The listing builds one solid part. Answer for the finished solid, in the listing's coordinates (mm). Coordinates: 2 decimals unless noted, no trailing zeros. Order: outer loops, then holes, each group sorted by start corner. A loop starts at its lowest first (then second) coordinate and runs counter-clockwise, first axis right, second up. Notation, with made-up numbers: (-29, -39) -> (23, -39) arc R35 cw to (23, -3) -> close; hole circle Ø8 at (-37, -37.5). An arc over 180 degrees is marked (long way). Return JSON: item names as keys, results as strings.
from build123d import *

# Parameters (mm, degrees)
F1_DEPTH = 6.5
F3_DEPTH = 80


with BuildPart() as f1:
    # F0 (on Front) → F1 (new body, symmetric)
    with BuildSketch(Plane.XZ):
        Polygon((80, 0), (0, 0), (0, -20), (80, -5), align=None)
    extrude(amount=F1_DEPTH, both=True)

    # F2 (on Right) → F3 (intersect)
    with BuildSketch(Plane.YZ):
        with BuildLine():
            Line((6.5, 0), (-6.5, 0))
            Line((-6.5, 0), (-6.5, -5))
            ThreePointArc((-6.5, -5), (-2.782918, -12.094306), (-1.5, -20))
            Line((-1.5, -20), (1.5, -20))
            ThreePointArc((1.5, -20), (2.782918, -12.094306), (6.5, -5))
            Line((6.5, -5), (6.5, 0))
        make_face()
    extrude(amount=F3_DEPTH, mode=Mode.INTERSECT)


solid = f1.part
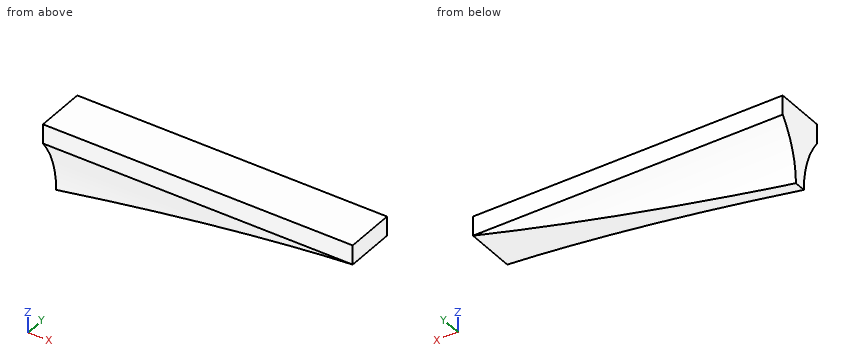
1. The part is cut by section B-B on x = 48. Give the vertices of the cut face in (y, z).
Answer block:
{"outline": "(-6.5, -5) arc R25 cw to (-3.18, -11) -> (3.18, -11) arc R25 cw to (6.5, -5) -> (6.5, 0) -> (-6.5, 0) -> close"}
2. The part is cut by section D-D on y = 5.5. Give the vertices of the cut face in (x, z).
Answer block:
{"outline": "(0, -6.44) -> (72.34, -6.44) -> (80, -5) -> (80, 0) -> (0, 0) -> close"}
3. Consider line 1 (Z direction, x = 22, y = -4); line 2 (Z direction, x = 36, y = 3.5); line 3 (Y direction, x = 12, z = -9.5). Determine where each line is inside the solid, lowest interval first. Write a range as from..to.
Answer block:
{"line 1": "z = -9.1..0", "line 2": "z = -10.2..0", "line 3": "y = -3.81..3.81"}
4. Each of these flat-tipped pins is pushed along its axis until it touches: pin 1 Ø10 at (x, z) = (11.5, -18) entering from +Y; pin 2 Ø1.5 at (y, z) = (-3.5, -12.5) entering from +X; pin 3 Ø1 at (x, y) = (51.5, 3) entering from -Z. Where does it stop, or does it pass through?
Answer block:
{"pin 1": "stops at y = 2.5", "pin 2": "passes through", "pin 3": "stops at z = -10.44"}
5. The part is cut by section A-A on y = 2.5. Give the vertices of the cut face in (x, z).
Answer block:
{"outline": "(0, -13) -> (37.33, -13) -> (80, -5) -> (80, 0) -> (0, 0) -> close"}
6. The part is cut by section C-C on z = -15. Give the vertices of the cut face in (x, y).
Answer block:
{"outline": "(0, -2.01) -> (26.67, -2.01) -> (26.67, 2.01) -> (0, 2.01) -> close"}
